Design review of the part built by this model. Coordinates are the model's own, in mm. Coordinates: 2 decimals unless noted, no trailing zeros. Write each loop counter-clockwise with the first axis right and the second up, starting at its lowest first coordinate (ties: lowest second). Pieces come first, ordered by that corner, then holes. Notation, with made-up numbers: (-31.5, -31) -> (-8.5, -31) arc R13 cw to (-8.5, -16) -> close; hole circle Ø11 at (-35, 53.25). An arc over 180 degrees is marked (long way). One line per question, with ' | ' between items. Start each with the question number.
Q1. Wall thickness on probe 1 along Y at (x, z) = (75.5, 4.6): over which ranges is the line inside the solid? List them lowest first.
Q2. Add section B-B on y = 6.25. Give the number of separate pieces and of enclosed holes in the cut face, and give its area (3 significant figures).
Q3. For P1, Ø5, axis at x = 52.5, y = 6, coming from the +Z side, flat-tipped, find the tip position at first contact; note if it passes through.
Q4. Add section A-A on x = 41. State the section outline as (y, z) points.
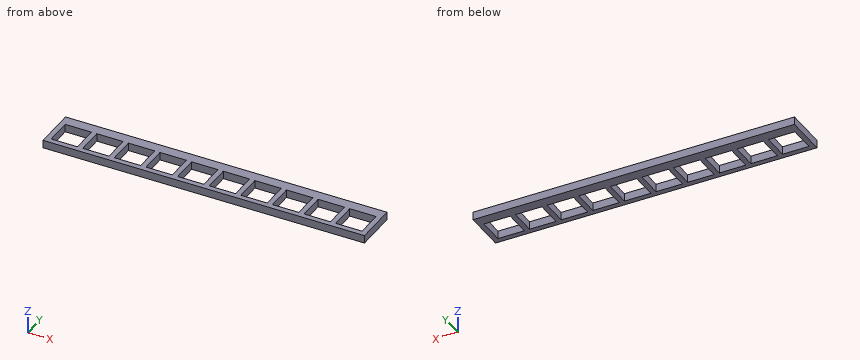
from build123d import *

# Parameters (mm, degrees)
BOX_W         = 10
BOX_H         = 10
BOX_DEPTH     = 10
ARRAY_X_COUNT = 10
ARRAY_X_PITCH = 12
BOX001_W      = 122
BOX001_H      = 16
BOX001_DEPTH  = 3


with BuildPart() as array:
    # Box → Box (new body)
    with BuildSketch(Plane.XY):
        with Locations((5, 5)):
            Rectangle(BOX_W, BOX_H)
    extrude(amount=BOX_DEPTH)

    # Array X: Array ×10


with BuildPart() as array_1:
    add(array.part)
    with Locations(*[(i * ARRAY_X_PITCH, 0, 0) for i in range(1, ARRAY_X_COUNT)]):
        add(array.part)


with BuildPart() as cut:
    # Box001 → Box001 (new body)
    with BuildSketch(Plane(origin=(-2, -2, 4), x_dir=(1, 0, 0), z_dir=(0, 0, 1))):
        with Locations((61, 8)):
            Rectangle(BOX001_W, BOX001_H)
    extrude(amount=BOX001_DEPTH)

    # Cut: cut Array
    add(array_1.part, mode=Mode.SUBTRACT)


solid = cut.part
Output values:
1) probe 1: y = -2 to 0, 10 to 14
2) separate pieces: 11 | enclosed holes: 0 | area: 66.0 mm2
3) P1: passes through
4) outline: (-2, 4) -> (0, 4) -> (0, 7) -> (-2, 7) -> close; (10, 4) -> (14, 4) -> (14, 7) -> (10, 7) -> close
